Autodesk Inventor part; units mm, degrees
ref_plane "YZ Plane" through (0, 0, 0) normal (1, 0, 0) x (0, 1, 0)
ref_plane "XZ Plane" through (0, 0, 0) normal (0, 1, 0) x (-1, 0, 0)
ref_plane "XY Plane" through (0, 0, 0) normal (0, 0, 1) x (1, 0, 0)
sketch "Sketch1" plane through (0, 0, 0) normal (0, 0, 1) x (1, 0, 0)
  line L0 (0, 0) -> (50.8, 0)
  line L1 (50.8, 0) -> (50.8, 25.4)
  line L2 (50.8, 25.4) -> (0, 25.4)
  line L3 (0, 25.4) -> (0, 0)
  line L4 (3.175, 3.175) -> (47.625, 3.175)
  line L5 (47.625, 3.175) -> (47.625, 22.225)
  line L6 (47.625, 22.225) -> (3.175, 22.225)
  line L7 (3.175, 22.225) -> (3.175, 3.175)
  dimension "d0" = 25.4
  dimension "d1" = 50.8
  dimension "d2" = 3.175
  dimension "d3" = 3.175
  dimension "d4" = 3.175
  dimension "d5" = 3.175
extrude "Extrusion1" add sketch "Sketch1" along normal blind 254
sketch "Sketch2" plane through (50.8, 0, 0) normal (1, 0, 0) x (0, 0, -1)
  line L0 (-254, 25.4) -> (-254, 0)
  line L1 (0, 0) -> (-254, 0)
  line L2 (0, 0) -> (0, 25.4)
  line L3 (0, 25.4) -> (-254, 25.4)
  circle A0 centre (-241.3, 12.7) radius 4.7625
  arc A1 (-241.3, 25.4) -> (-241.3, 0) centre (-241.3, 12.7) ccw
  dimension "d8" = 9.525
  dimension "d9" = 12.7
extrude "Extrusion2" cut sketch "Sketch2" against normal blind 254 contours L3 A1 L0 | A1 L1 L0 | A0
equation "\"d2\" = d5"
equation "\"d3\" = d2"
equation "\"d4\" = d3"
properties part number "apendage arm"
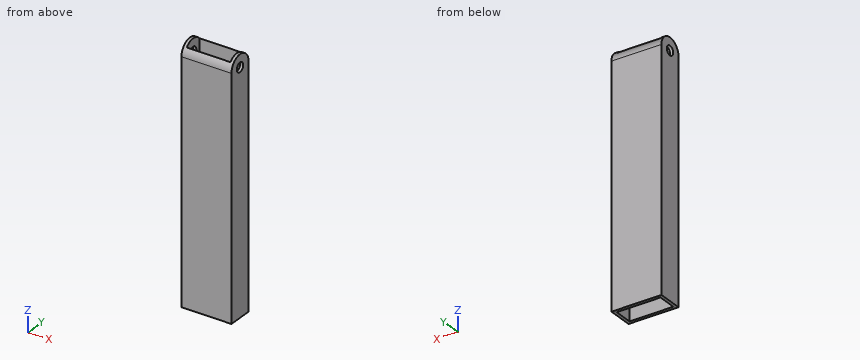
Can you work these out from the model? Positions are in its coordinate system, mm. Round coordinates to 2 decimals unless told otherwise and drop trailing zeros. Write each loop counter-clockwise with the first axis right and the second up, starting at its lowest first coordinate (ties: lowest second). Pieces come first, ordered by that corner, then holes. Notation, with made-up numbers: (38.5, 55.5) - (87.5, 55.5) arc R14 cw to (87.5, 73.5) - close; hole circle Ø8 at (23.25, -19). An arc over 180 degrees is marked (long way). Write each question's results on one line, items separated by ' | '. Start each with the question number.
1) Suppose I cut it at C-C (y = 12.7). List the corners of the cut face in (x, z) for me (1 decimal), and give its area (3 significant figures).
2) For pin 1 Ø8.5 at (y, z) = (12.7, 241.3) entering from +X; pin 2 Ø12.5 at (y, z) = (12.7, 241.3) entering from -X, each with a flat end and sliding along its axis, tell me the tip position at first contact or that it passes through.
3) Please list where these lines run through material, in increasing order: line 1 (Y direction, x = 11, z = 102) (3 decimals); line 2 (X direction, y = 18.5, z = 38) (3 decimals); line 3 (Y direction, x = 2.1, z = 241.3).
4) Suppose I cut it at A-A (x = 30). List the corners of the cut face in (y, z) for me (3 decimals).
5) Suppose I cut it at B-B (z = 150). List the corners of the cut face in (x, y) for me (3 decimals).
Here are the results:
1) outline: (0, 0) - (3.2, 0) - (3.2, 236.5) - (0, 236.5) - close; (0, 246.1) - (3.2, 246.1) - (3.2, 254) - (0, 254) - close; (47.6, 0) - (50.8, 0) - (50.8, 236.5) - (47.6, 236.5) - close; (47.6, 246.1) - (50.8, 246.1) - (50.8, 254) - (47.6, 254) - close | area: 1,550 mm2
2) pin 1: passes through | pin 2: stops at x = 0
3) line 1: y = 0 to 3.175, 22.225 to 25.4 | line 2: x = 0 to 3.175, 47.625 to 50.8 | line 3: y = 0 to 7.94, 17.46 to 25.4
4) outline: (0, 0) - (3.175, 0) - (3.175, 249.7) arc R12.7 ccw to (0, 241.3) - close; (22.225, 0) - (25.4, 0) - (25.4, 241.3) arc R12.7 ccw to (22.225, 249.7) - close
5) outline: (0, 0) - (50.8, 0) - (50.8, 25.4) - (0, 25.4) - close; hole (3.175, 3.175) - (47.625, 3.175) - (47.625, 22.225) - (3.175, 22.225) - close
